from build123d import *

# Parameters (mm, degrees)
BOSS_EXTRUDE1_DEPTH = 7
SKETCH2_R           = 2.5
SKETCH2_R_2         = 9
SKETCH2_R_3         = 8
BOSS_EXTRUDE2_DEPTH = 20
FILLET1_R           = 1
SCALE1_SCALE        = 5


with BuildPart() as part:
    # Sketch1 → Boss-Extrude1 (new body)
    with BuildSketch(Plane(origin=(0, 0, 0), x_dir=(1, 0, 0), z_dir=(0, 1, 0))):
        with BuildLine():
            Line((-61.391033774, -32.868924483), (25.33933743, -32.868924483))
            ThreePointArc((25.33933743, -32.868924483), (32.410405242, -29.939992295), (35.33933743, -22.868924483))
            Line((35.33933743, -22.868924483), (35.33933743, -2.779955787))
            ThreePointArc((35.33933743, -2.779955787), (32.410405242, 4.291112025), (25.33933743, 7.220044213))
            Line((25.33933743, 7.220044213), (-61.391033774, 7.220044213))
            ThreePointArc((-61.391033774, 7.220044213), (-68.462101586, 4.291112025), (-71.391033774, -2.779955787))
            Line((-71.391033774, -2.779955787), (-71.391033774, -22.868924483))
            ThreePointArc((-71.391033774, -22.868924483), (-68.462101586, -29.939992295), (-61.391033774, -32.868924483))
        make_face()
    extrude(amount=BOSS_EXTRUDE1_DEPTH)

    # Sketch2 → Boss-Extrude2 (add)
    # profile 1 of 2: a face of its own
    with BuildSketch(Plane(origin=(0, 7, 0), x_dir=(1, 0, 0), z_dir=(0, 1, 0))):
        with Locations(Location((-43.693698634, -12.824440135, 0), (0, 0, 270))):
            Circle(SKETCH2_R)
    # profile 2 of 2: a face of its own
    with BuildSketch(Plane(origin=(0, 7, 0), x_dir=(1, 0, 0), z_dir=(0, 1, 0))):
        with Locations(Location((9.591521865, -12.824440135, 0), (0, 0, 270))):
            Circle(SKETCH2_R_2)
        with Locations(Location((9.591521865, -12.824440135, 0), (0, 0, 270))):
            Circle(SKETCH2_R_3, mode=Mode.SUBTRACT)
    extrude(amount=BOSS_EXTRUDE2_DEPTH)

    # Fillet1
    fillet1_edges = [part.edges().sort_by_distance(p)[0] for p in [
        (-43.693698634, 7, 10.324440135),
        (9.591521865, 7, 3.824440135),
    ]]
    fillet(fillet1_edges, radius=FILLET1_R)


with BuildPart() as part_1:
    # Scale1: scaled about (0, 0, 0)
    add(part.part.scale(SCALE1_SCALE))


solid = part_1.part
For this review, take the finished solid that the model builds, in its own axes (mm). A direction names the side the tool comes from. Round coordinates to 2 decimals unless told otherwise and drop trailing zeros. Write each loop counter-clockwise with the first axis right and the second up, starting at its lowest first coordinate (ties: lowest second). Pieces come first, ordered by that corner, then holes. Notation, with made-up numbers: (-27.75, -36) - (28.25, -36) arc R17 cw to (28.25, -32) - close; hole circle Ø11 at (62, 16). An arc over 180 degrees is marked (long way). Write item = value, one per line. Start each with the question number.
1. Draft analysis for pull direction Z (two halves, no side actions). For faces 1 (the face through (-93, 17, 164.345)), 2 (the face through (-94, 0, 63)), 3 (the face through (59.973, 84.3, 102.275)), state which applies: released by +Z, released by -Z, zero draft, split by the parting line, or undercut.
2. Consider section C-C on x = -99. State the section outline as (y, z) points, plus the area to 3 significant figures.
3. Wall thickness on L1, parallel to Z at x = 50, y = 124.5; L2, parallel to Y at x = -261, z = -14.5; L3, parallel to Z at x = 6.5, y = 45: over which ranges is each line inside the solid? List them lowest first.
4. For faces 4 (the face through (47, 35, 64)), 5 (the face through (-218, 135, 64)), list the 3-axis set-ups (+Z, -Z, +X, -X, +Y, -Y) from which the entire face can be reached by the end or side of a thin tool; tool diameter is ignored.
5. For pin 1 Ø3 at (x, z) = (-194, -2) entering from -Y; pin 2 Ø1 at (x, y) = (-223, 56.5) entering from -Z; pin 3 Ø1 at (x, z) = (34, 115.5) entering from +Y; pin 4 Ø5 at (y, z) = (87, 89) entering from +X, all flat-tipped, find the tip position at first contact; note any pin that passes through.
6. Consider section A-A on y = 51. State the section outline as (x, z) points, plus the area to 3 significant figures.
7. Consider section D-D on z = -18. State the section outline as (x, y) points.
8. Consider section B-B on y = 9. State the section outline as (x, z) points.
Evaluation:
q1.face_1 = released by +Z
q1.face_2 = zero draft
q1.face_3 = undercut
q2.outline = (0, -36.1) - (35, -36.1) - (35, 164.34) - (0, 164.34) - close
q2.area = 7,020 mm2
q3.L1 = 19.17 to 24.17, 104.07 to 109.08
q3.L2 = 0 to 35
q3.L3 = 46.62 to 81.62
q4.face_4 = +Y
q4.face_5 = +Z, -Z, +X, -X, +Y
q5.pin_1 = 0
q5.pin_2 = 52.29
q5.pin_3 = 35
q5.pin_4 = 87
q6.outline = circle Ø25 at (-218.47, 64.12); circle Ø90 at (47.96, 64.12); hole circle Ø80 at (47.96, 64.12)
q6.area = 1,830 mm2
q7.outline = (-345.46, 0) - (165.2, 0) - (165.2, 35) - (-345.46, 35) - close
q8.outline = (-356.96, 13.9) arc R50 ccw to (-306.96, -36.1) - (126.7, -36.1) arc R50 ccw to (176.7, 13.9) - (176.7, 114.34) arc R50 ccw to (126.7, 164.34) - (-306.96, 164.34) arc R50 ccw to (-356.96, 114.34) - close
